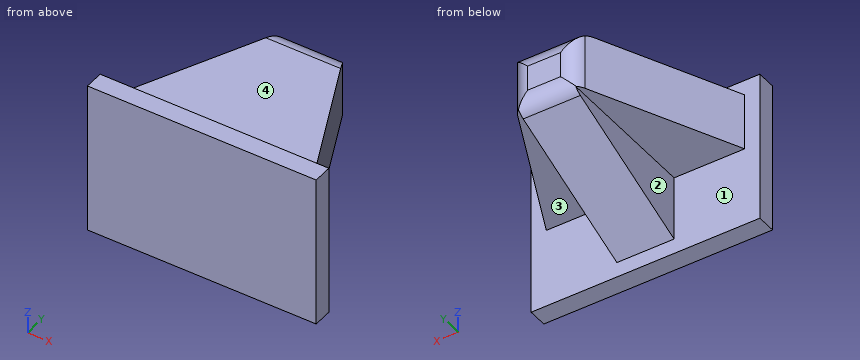
from build123d import *

# Parameters (mm, degrees)
SKETCH1_W               = 38.1
SKETCH1_H               = 25.4
SKETCH1_W_2             = 33.02
SKETCH1_H_2             = 20.32
SKETCH1_W_3             = 11.7475
SKETCH1_H_3             = 10.795
SKETCH1_W_4             = 9.525
BOSS_EXTRUDE1_DEPTH     = 3.175
SKETCH1_3_W             = 9.525
SKETCH1_3_H             = 10.795
BOSS_EXTRUDE2_DEPTH     = 25.4
CUT_EXTRUDE1_DEPTH      = 40.123421374
CUT_EXTRUDE2_DEPTH      = 38.060560658
CUT_EXTRUDE2_DEPTH_BACK = 38.060560658
FILLET7_R               = 3.175


with BuildPart() as part:
    # Sketch1 → Boss-Extrude1 (new body)
    # profile 1 of 5: a face of its own
    with BuildSketch(Plane(origin=(0, 0, 0), x_dir=(1, 0, 0), z_dir=(0, 1, 0))):
        Rectangle(SKETCH1_W, SKETCH1_H)
        Rectangle(SKETCH1_W_2, SKETCH1_H_2, mode=Mode.SUBTRACT)
    # profile 2 of 5: a face of its own
    with BuildSketch(Plane(origin=(0, 0, 0), x_dir=(1, 0, 0), z_dir=(0, 1, 0))):
        with Locations((-10.63625, 4.7625)):
            Rectangle(SKETCH1_W_3, SKETCH1_H_3)
    # profile 3 of 5: a face of its own
    with BuildSketch(Plane(origin=(0, 0, 0), x_dir=(1, 0, 0), z_dir=(0, 1, 0))):
        with Locations((10.63625, 4.7625)):
            Rectangle(SKETCH1_W_3, SKETCH1_H_3)
    # profile 4 of 5: a face of its own
    with BuildSketch(Plane(origin=(0, 0, 0), x_dir=(1, 0, 0), z_dir=(0, 1, 0))):
        with Locations((0, 4.7625)):
            Rectangle(SKETCH1_W_4, SKETCH1_H_3)
    # profile 5 of 5: a face of its own
    with BuildSketch(Plane(origin=(0, 0, 0), x_dir=(1, 0, 0), z_dir=(0, 1, 0))):
        Polygon((-4.7625, -0.635), (-16.51, -0.635), (-16.51, -10.16), (16.51, -10.16), (16.51, -0.635), (4.7625, -0.635), align=None)
    extrude(amount=-BOSS_EXTRUDE1_DEPTH)

    # Sketch1<3> → Boss-Extrude2 (add)
    with BuildSketch(Plane(origin=(0, 0, 0), x_dir=(1, 0, 0), z_dir=(0, 1, 0))):
        with Locations((0, 4.7625)):
            Rectangle(SKETCH1_3_W, SKETCH1_3_H)
        Polygon((-4.7625, -0.635), (-16.51, -0.635), (-16.51, -10.16), (16.51, -10.16), (16.51, -0.635), (4.7625, -0.635), align=None)
    extrude(amount=BOSS_EXTRUDE2_DEPTH)

    # Sketch2 → Cut-Extrude1 (cut, through all)
    with BuildSketch(Plane.XY.offset(10.16)):
        Polygon((-16.51, 25.4), (-16.51, 0), (-4.7625, 25.4), align=None)
        Polygon((4.7625, 25.4), (16.51, 0), (16.51, 25.4), align=None)
    extrude(amount=-CUT_EXTRUDE1_DEPTH, mode=Mode.SUBTRACT)

    # Sketch3 → Cut-Extrude2 (cut, two sides: drawn at the far end of the back side and taken through both)
    with BuildSketch(Plane(origin=(4.7625, 0, 0), x_dir=(0, 0, -1), z_dir=(1, 0, 0)).offset(-CUT_EXTRUDE2_DEPTH_BACK)):
        Polygon((-0.635, 25.4), (10.16, 0), (10.16, 25.4), align=None)
    extrude(amount=CUT_EXTRUDE2_DEPTH + CUT_EXTRUDE2_DEPTH_BACK, mode=Mode.SUBTRACT)

    # Fillet7
    # the kernel refuses this fillet: 3.175 mm, written as the material it takes off along each edge
    with BuildSketch(Plane(origin=(-12.7, 25.4, 10.16), x_dir=(0, 0, -1), z_dir=(1, 0, 0))) as fillet7_piece_1:
        with BuildLine():
            CenterArc((FILLET7_R, -FILLET7_R), FILLET7_R, 90, 90)
            Line((0, -FILLET7_R), (0, 0))
            Line((0, 0), (FILLET7_R, 0))
        make_face()
    extrude(amount=25.4, mode=Mode.SUBTRACT)
    with BuildSketch(Plane(origin=(-4.7625, 25.4, 15.234238466), x_dir=(1, 0, 0), z_dir=(0, 0, -1)), Plane(origin=(4.7625, 25.4, 15.234238466), x_dir=(0.4197775063604339, -0.9076270407793146, 0), z_dir=(0, 0, -1))) as fillet7_piece_2:
        with BuildLine():
            CenterArc((FILLET7_R * 0.639274137471, FILLET7_R), FILLET7_R, 204.820541335, 65.179458665)
            Line((-FILLET7_R * 0.268352903308, FILLET7_R * 0.58022249364), (0, 0))
            Line((0, 0), (FILLET7_R * 0.639274137471, 0))
        make_face()
    extrude(amount=19.673476932, mode=Mode.SUBTRACT)
    with BuildSketch(Plane(origin=(10.013677669, 25.4, 0.635), x_dir=(0, 0, 1), z_dir=(-1, 0, 0))) as fillet7_piece_3:
        with BuildLine():
            CenterArc((FILLET7_R * 0.661565690605, -FILLET7_R), FILLET7_R, 90, 66.974507991)
            Line((-FILLET7_R * 0.258765227853, -FILLET7_R * 0.608859359655), (0, 0))
            Line((0, 0), (FILLET7_R * 0.661565690605, 0))
        make_face()
    extrude(amount=20.027355338, mode=Mode.SUBTRACT)


solid = part.part
Check sheet for the modelled part. Datum: model origin and axes. Units: mm. Face numbers are marked on the shaded views. A direction names the side the tool comes from. Round coordinates to 2 decimals unless told otherwise and drop trailing zeros. Order: outer loops, then holes, each group sorted by start corner. A loop starts at its lowest first (then second) coordinate and runs counter-clockwise, first axis right, second up.
Q1. Depth check by flat-ended pin: P1, Ø11, axis at x = 8, y = 11, coming from the +Z side; P2, Ø6, axis at x = 1.5, y = 0.5, coming from the -Z side; P3, Ø1.5, axis at y = 6.5, z = 5.5, coming from the +X side; P4, Ø12, axis at y = 18, z = -1.5, coming from the +X side. Enter the tip coordinate at first touch or a pass-through.
Filled sheet:
P1: stops at z = 10.16
P2: stops at z = -12.7
P3: stops at x = 13.85
P4: stops at x = 10.78
Q2. Cross-section at B-B, the plane y = 0.5. Enter the section's corners in (x, z) (1 decimal).
Filled sheet:
outline: (-16.3, 0.6) - (-4.8, 0.6) - (-4.8, -9.9) - (4.8, -9.9) - (4.8, 0.6) - (16.3, 0.6) - (16.3, 10.2) - (-16.3, 10.2) - close
Q3. Scan lines: L1, parallel to Y at x = 10, z = -8 (3 decimals); L2, parallel to Z at x = -12, y = 9 (3 decimals); L3, parallel to X at y = 4.75, z = -6. Record each from-to range of solid material in increasing order.
Filled sheet:
L1: y = -3.175 to 0
L2: z = 0.635 to 10.16
L3: x = -4.76 to 4.76
Q4. Cross-section at A-A, the plane z = 6. Enter the section's corners in (x, y) (3 decimals), plus the area to 3 significant figures.
Filled sheet:
outline: (-19.05, -3.175) - (19.05, -3.175) - (19.05, 0) - (16.51, 0) - (5.615, 23.558) arc R3.175 ccw to (2.733, 25.4) - (-2.733, 25.4) arc R3.175 ccw to (-5.615, 23.558) - (-16.51, 0) - (-19.05, 0) - close
area: 660 mm2
Q5. Cross-section at C-C, the plane x = 2. Enter the section's corners in (y, z) (3 decimals), plus the area to 3 significant figures.
Filled sheet:
outline: (-3.175, -12.7) - (0, -12.7) - (0, -10.16) - (23.467, -0.187) arc R3.175 ccw to (25.4, 2.735) - (25.4, 6.985) arc R3.175 ccw to (22.225, 10.16) - (0, 10.16) - (0, 12.7) - (-3.175, 12.7) - close
area: 457 mm2
Q6. Set-up check for the marked faces 1, 2, 3 and 4: record each of +Z, -Z, +X, -X, +Y, -Y from which the full face is reachable in a straight line by a thin tool's end or side.
Filled sheet:
face 1: +Y
face 2: -Z, -X, +Y
face 3: -Z, +X, +Y
face 4: +Z, +X, -X, +Y
